Check sheet for the modelled part. Datum: model origin and axes. Units: mm. Face numbers are marked on the shaded views. Round coordinates to 2 decimals unless told otherwise and drop trailing zeros. Loops run counter-clockwise (first coordinate to the right, second up) from the corner with the lowest first, then second, coordinate; pieces in that order, holes last. Notation, with made-up numbers: M 74,-3 L 130,-3 A14 cw 130,16 Z; hole C 84.5,-20.5 d5. An arc over 180 degrees is marked long. Write item = value, one per line. Start each with the question number.
(1) Go/stop test with flat-tipped pins: P1, Ø2, axis at x = -12.5, y = 1, coming from the +Z side; P2, Ø2, axis at y = 3.5, z = -12, coming from the -X side; P3, Ø8, axis at x = -18.5, z = 8, coming from the +Y side; P4, Ø1.5, axis at y = 1.5, z = 0.5, coming from the -X side. Record where each tip stops, or that it passes through.
(2) Scan lines: L1, parallel to Z at x = 4, y = 0.95; L2, parallel to Z at x = -1.5, y = 0.9; L3, parallel to X at y = 4.45, z = 12. Record each from-to range of solid material in increasing order. Write a range as from..to.
(3) Mould release check, pull along Z, two halves, no side actions. Record for the marked faces 1, 2 and 3: pulls with the +Z half, pulls with the -Z half, needs draft (parallel to the pull), parting line crosses it, or undercut.
(4) Cross-section at B-B on x = 4. State how many separate pieces and enclosed holes the cut face has, plus the area to 3 significant figures.
(5) Cross-section at A-A on z = 8. Record the boundary of the cut face in (x, y), plus the area to 3 significant figures.
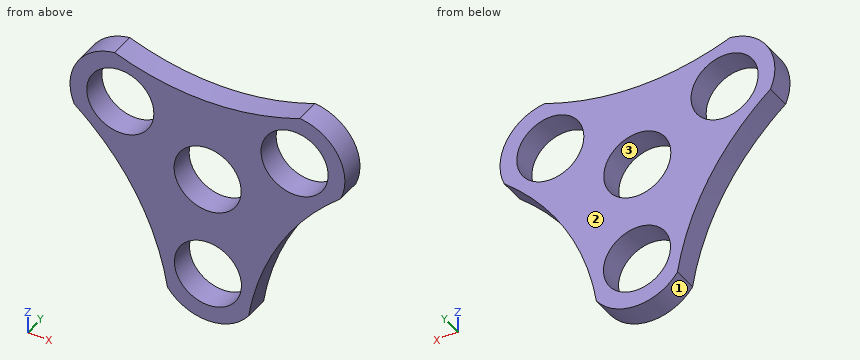
from build123d import *

# Parameters (mm, degrees)
SKETCH2_R           = 6.35
BOSS_EXTRUDE1_DEPTH = 4.7625


with BuildPart() as part:
    # Sketch2 → Boss-Extrude1 (new body)
    with BuildSketch(Plane(origin=(0, 0, 0), x_dir=(1, 0, 0), z_dir=(0, 1, 0))):
        with BuildLine():
            ThreePointArc((7.763480479, 24.65151799), (0.088455744, 28.574863042), (-7.61008297, 24.69786127))
            add(Edge.make_bspline(
                [(-7.61008297, 24.69786127), (-9.592104105, 12.649393813), (-15.73585932, 2.097225899), (-25.22422914, -5.588137723)],
                knots=[0, 0, 0, 0, 1, 1, 1, 1], degree=3))
            ThreePointArc((-25.22422914, -5.588137723), (-24.792958655, -14.207033662), (-17.57711737, -18.940213988))
            add(Edge.make_bspline(
                [(-17.57711737, -18.940213988), (-6.152008529, -14.631981889), (6.058316415, -14.676034081), (17.458404858, -19.050043608)],
                knots=[0, 0, 0, 0, 1, 1, 1, 1], degree=3))
            ThreePointArc((17.458404858, -19.050043608), (24.704052244, -14.361071884), (25.187751026, -5.744117819))
            add(Edge.make_bspline(
                [(25.187751026, -5.744117819), (15.743744455, 1.995695857), (9.676165927, 12.591849246), (7.763480479, 24.65151799)],
                knots=[0, 0, 0, 0, 1, 1, 1, 1], degree=3))
        make_face()
        with Locations(Location((0, 0, 0), (0, 0, 90))):
            Circle(SKETCH2_R, mode=Mode.SUBTRACT)
        with Locations(Location((0.059742965, 19.049906319, 0), (0, 0, 90))):
            Circle(SKETCH2_R, mode=Mode.SUBTRACT)
        with Locations(Location((16.46783133, -9.576692085, 0), (0, 0, 90))):
            Circle(SKETCH2_R, mode=Mode.SUBTRACT)
        with Locations(Location((-16.527574295, -9.473214235, 0), (0, 0, 90))):
            Circle(SKETCH2_R, mode=Mode.SUBTRACT)
    extrude(amount=BOSS_EXTRUDE1_DEPTH)


solid = part.part
Result:
q1.P1 = 17.6
q1.P2 = -11.96
q1.P3 = 4.76
q1.P4 = -20.51
q2.L1 = -27.72..-24.03, -14.07..-4.93, 4.93..15.92
q2.L2 = -28.45..-25.21, -12.89..-6.17, 6.17..15.76
q2.L3 = -25.71..-22.35, -10.7..10.6, 22.34..25.68
q3.face_1 = pulls with the -Z half
q3.face_2 = needs draft
q3.face_3 = undercut
q4.separate_pieces = 3
q4.enclosed_holes = 0
q4.area = 113 mm^2
q5.outline = M -25.94,0 L -22.7,0 L -22.7,4.76 L -25.94,4.76 Z; M -10.35,0 L 10.32,0 L 10.32,4.76 L -10.35,4.76 Z; M 22.62,0 L 25.86,0 L 25.86,4.76 L 22.62,4.76 Z
q5.area = 129 mm^2
